For this review, take the finished solid that the model builds, in its own axes (mm). A direction names the side the tool comes from. Coordinates: 2 decimals unless noted, no trailing zeros. Write each loop counter-clockwise with the first axis right and the second up, starting at its lowest first coordinate (ties: lowest second). Pieces come first, ordered by that corner, then holes.
```python
from build123d import *

# Parameters (mm, degrees)
F1_DEPTH = 5
F2_ANGLE = 90


with BuildPart() as f1:
    # F0 (on Front) → F1 (new body, symmetric)
    with BuildSketch(Plane.XZ):
        with BuildLine():
            Line((273, 36), (0, 18.6097864581))
            Line((0, 18.6097864581), (-10.1442882229, 17.9635910793))
            ThreePointArc((-10.1442882229, 17.9635910793), (-26.9908954672, -0.5724336526), (-9, -18))
            Line((-9, -18), (265, -18))
            add(Edge.make_bspline(
                [(265, -18), (310, -18), (406.8679036126, -46.6311179489), (489.31460039, -164.7387197182), (468.8864991068, -212.4993609156), (466.5754698987, -216.9332242423)],
                knots=[0, 0, 0, 0, 0.3972155542, 0.7825964326, 1, 1, 1, 1], degree=3))
            ThreePointArc((466.5754698987, -216.9332242423), (472.8213356215, -214.1061695722), (477.0533174327, -219.5))
            ThreePointArc((477.0533174327, -219.5), (475.8300498393, -222.9770681469), (472.6991622653, -224.9223006529))
            Line((472.6991622653, -224.9223006529), (481.7930329869, -222.9111561664))
            Line((481.7930329869, -222.9111561664), (541.3538880895, -209.7390439802))
            Line((541.3538880895, -209.7390439802), (556, -206.5))
            add(Edge.make_bspline(
                [(435, 0), (456.9281394948, -12.0065273205), (545.1260274002, -66.7040872695), (566.7745237898, -163.0993973046), (559.2541435751, -191.8572355891), (556, -206.5)],
                knots=[0, 0, 0, 0, 0.4044974221, 0.7598198092, 1, 1, 1, 1], degree=3))
            ThreePointArc((435, 0), (356.5575563064, 29.5090033787), (273, 36))
        make_face()
        with BuildLine():
            Line((6.5, -6), (-6.5, -6))
            ThreePointArc((-6.5, -6), (-12.5, 0), (-6.5, 6))
            Line((-6.5, 6), (0, 6))
            Line((0, 6), (6.5, 6))
            ThreePointArc((6.5, 6), (12.5, 0), (6.5, -6))
        make_face(mode=Mode.SUBTRACT)
        with BuildLine():
            ThreePointArc((477.0533174327, -219.5), (472.8213356215, -214.1061695722), (466.5754698987, -216.9332242423))
            ThreePointArc((466.5754698987, -216.9332242423), (467.0925146794, -222.8783735224), (472.6991622653, -224.9223006529))
            ThreePointArc((472.6991622653, -224.9223006529), (475.8300498393, -222.9770681469), (477.0533174327, -219.5))
        make_face()
        Polygon((554.741936541, -270.2763065435), (541.3538880895, -209.7390439802), (481.7930329869, -222.9111561664), (495.1810814384, -283.4484187297), (515.2443770491, -286.180481913), align=None)
    extrude(amount=F1_DEPTH, both=True)


with BuildPart() as f1_1:
    # F2: moved
    add(f1.part.rotate(Axis((0, 0, 97.4653586745), (0, 0, 1)), F2_ANGLE))

    # F4 (on face) → F5 section 0
    with BuildSketch(Plane(origin=(0, 171.0419719317, -424.7777897972), x_dir=(1, 0, 0), z_dir=(0, 0.3735186178, -0.9276226831)), mode=Mode.PRIVATE) as f5_s0:
        with BuildLine():
            Line((-5, -371.0586334279), (5, -371.0586334279))
            ThreePointArc((5, -371.0586334279), (0, -366.0586334279), (-5, -371.0586334279))
        make_face()
    loft([f5_s0.sketch, Vertex(0, 317.4776060293, -259.2501448204)])


with BuildPart() as f1_2:
    # F6: moved
    add(f1_1.part.moved(Location((0, -350, 48))))


with BuildPart() as f1_3:
    # F7: moved
    add(f1_2.part.moved(Location((-30, 0, 0))))


solid = f1_3.part
```
Q1. Tool access review of faces 1 (the flat face through (-35, 6, 20)), 2 (the flat face through (-29.93, 138.393, -204.756)), 3 (the flat face through (-29.93, 198.14, -192.43)): name each direction out of +Z, -Z, +X, -X, +Y, -Y from which nothing blocks a thin tool from reaching the whole face with its end or side.
Ans:
face 1: +Z, -Z, -X, +Y, -Y
face 2: +X, -X
face 3: +X, -X, +Y
Q2. For probe 1 along Z at (x, y) = (-32, 55.5); probe 2 along Z at (x, y) = (-32.5, -282); probe 3 along Y at (x, z) = (-28.75, -46), list the stretches that pass through material, from the lowest coordinate up.
Ans:
probe 1: z = -223.75 to -223.24, -19.81 to 62.11
probe 2: z = 30 to 70.94
probe 3: y = 82.94 to 192.72
Q3. Add section B-B (y = -280.5). State the section outline as (x, z) points, then the cut area to 3 significant figures.
Ans:
outline: (-35, 30) - (-25, 30) - (-25, 71.04) - (-35, 71.04) - close
area: 410 mm2
Q4. Clearance check with flat-ended pins moving along their axes: pin 1 Ø3 at (x, y) = (-31, -348.5) entering from +Z; pin 2 Ø3 at (x, y) = (-28.5, -272.5) entering from -Z; pin 3 Ø2 at (x, y) = (-32.5, 23.5) entering from +Z. State where each tip first meets the part, or that it passes through.
Ans:
pin 1: stops at z = 66.8
pin 2: stops at z = 30
pin 3: stops at z = 73.5
Q5. Draft analysis for pull direction Z (two halves, no side actions). For faces 4 (the flat face through (-30.06, 74.83, -225.87)), 5 (the cylindrical face through (-30, -377, 48)), 6 (the cylindrical face through (-29.93, 7.71, 77.25)), state which applies: +Z half, -Z half, draft (parallel to the pull), parting line (faces both ways), or undercut.
Ans:
face 4: undercut
face 5: parting line
face 6: +Z half
Q6. Add section A-A (y = -220). State the section outline as (x, z) points.
Ans:
outline: (-35, 30) - (-25, 30) - (-25, 74.89) - (-35, 74.89) - close
